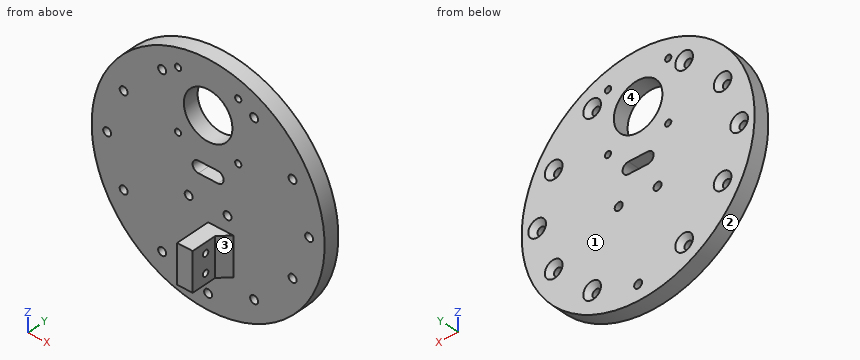
from build123d import *

# Parameters (mm, degrees)
SKETCH1_R                                           = 60
BOSS_EXTRUDE1_DEPTH                                 = 8
SKETCH2_R                                           = 12.5
SKETCH2_R_2                                         = 1.6
CUT_EXTRUDE1_DEPTH                                  = 86.229103011
SKETCH3_R                                           = 2.05
CUT_EXTRUDE2_DEPTH                                  = 86.229103011
CIRPATTERN1_COUNT                                   = 4
SKETCH4_R                                           = 2.05
CUT_EXTRUDE3_DEPTH                                  = 86.229103011
SKETCH5_R                                           = 2.05
CUT_EXTRUDE4_DEPTH                                  = 86.229103011
SKETCH6_W                                           = 8
SKETCH6_H                                           = 20
BOSS_EXTRUDE2_DEPTH                                 = 18
CHAMFER1_SIZE                                       = 5
SKETCH7_R                                           = 1.6
CUT_EXTRUDE5_DEPTH                                  = 93.455394651
CSK_FOR_M4_COUNTERSUNK_FLAT_HEAD_SCREW1_D           = 4.1
CSK_FOR_M4_COUNTERSUNK_FLAT_HEAD_SCREW1_DEPTH       = 7.999
CSK_FOR_M4_COUNTERSUNK_FLAT_HEAD_SCREW1_CSINK_D     = 9.1
CSK_FOR_M4_COUNTERSUNK_FLAT_HEAD_SCREW1_CSINK_ANGLE = 90
CSK_FOR_M4_COUNTERSUNK_FLAT_HEAD_SCREW1_TIP         = 1.231764269


with BuildPart() as part:
    # Sketch1 → Boss-Extrude1 (new body)
    with BuildSketch(Plane(origin=(0, 0, 0), x_dir=(1, 0, 0), z_dir=(0, 1, 0))):
        with Locations(Location((0, 0, 0), (0, 0, 270))):
            Circle(SKETCH1_R)
    extrude(amount=BOSS_EXTRUDE1_DEPTH)

    # Sketch2 → Cut-Extrude1 (cut, through all)
    with BuildSketch(Plane(origin=(0, 8, 0), x_dir=(1, 0, 0), z_dir=(0, 1, 0))):
        with Locations(Location((0, -33, 0), (0, 0, 270))):
            Circle(SKETCH2_R)
        with Locations(Location((-15.5, -48.5, 0), (0, 0, 270))):
            Circle(SKETCH2_R_2)
        with Locations(Location((15.5, -48.5, 0), (0, 0, 270))):
            Circle(SKETCH2_R_2)
        with Locations(Location((15.5, -17.5, 0), (0, 0, 270))):
            Circle(SKETCH2_R_2)
        with Locations(Location((-15.5, -17.5, 0), (0, 0, 270))):
            Circle(SKETCH2_R_2)
    extrude(amount=-CUT_EXTRUDE1_DEPTH, mode=Mode.SUBTRACT)

    # Sketch3 → Cut-Extrude2 (cut, through all)
    with BuildSketch(Plane(origin=(0, 8, 0), x_dir=(1, 0, 0), z_dir=(0, 1, 0))):
        with Locations(Location((-43.487067043, -23.68807717, 0), (0, 0, 270))):
            Circle(SKETCH3_R)
        with Locations(Location((-23.68807717, -43.487067043, 0), (0, 0, 270))):
            Circle(SKETCH3_R)
    cut_extrude2 = extrude(amount=-CUT_EXTRUDE2_DEPTH, mode=Mode.SUBTRACT)

    # CirPattern1: Cut-Extrude2 ×4 about axis
    cirpattern1_axis = Axis((0, 0, 0), (0, 1, 0))
    for i in range(1, CIRPATTERN1_COUNT):
        add(cut_extrude2.rotate(cirpattern1_axis, i * 360 / CIRPATTERN1_COUNT), mode=Mode.SUBTRACT)

    # Sketch4 → Cut-Extrude3 (cut, through all)
    with BuildSketch(Plane(origin=(0, 8, 0), x_dir=(1, 0, 0), z_dir=(0, 1, 0))):
        with Locations(Location((-52, 0, 0), (0, 0, 270))):
            Circle(SKETCH4_R)
        with Locations(Location((52, 0, 0), (0, 0, 270))):
            Circle(SKETCH4_R)
        with Locations(Location((0, 52, 0), (0, 0, 270))):
            Circle(SKETCH4_R)
    extrude(amount=-CUT_EXTRUDE3_DEPTH, mode=Mode.SUBTRACT)

    # Sketch5 → Cut-Extrude4 (cut, through all)
    with BuildSketch(Plane(origin=(0, 8, 0), x_dir=(1, 0, 0), z_dir=(0, 1, 0))):
        with Locations(Location((-10, 10, 0), (0, 0, 270))):
            Circle(SKETCH5_R)
        with Locations(Location((10, 10, 0), (0, 0, 270))):
            Circle(SKETCH5_R)
        with BuildLine():
            Line((-5, -3), (5, -3))
            ThreePointArc((5, -3), (8, -6), (5, -9))
            Line((5, -9), (-5, -9))
            ThreePointArc((-5, -9), (-8, -6), (-5, -3))
        make_face()
    extrude(amount=-CUT_EXTRUDE4_DEPTH, mode=Mode.SUBTRACT)

    # Sketch6 → Boss-Extrude2 (add)
    with BuildSketch(Plane.XZ):
        with Locations((4, -28)):
            Rectangle(SKETCH6_W, SKETCH6_H)
    extrude(amount=BOSS_EXTRUDE2_DEPTH)

    # Chamfer1
    chamfer1_edges = [part.edges().sort_by_distance(p)[0] for p in [
        (8, 0, -28),
    ]]
    chamfer(chamfer1_edges, length=CHAMFER1_SIZE)

    # Sketch7 → Cut-Extrude5 (cut, through all)
    with BuildSketch(Plane(origin=(8, 0, 0), x_dir=(0, 0, -1), z_dir=(1, 0, 0))):
        with Locations((23.25, -10.5)):
            Circle(SKETCH7_R)
        with Locations((32.75, -10.5)):
            Circle(SKETCH7_R)
    extrude(amount=-CUT_EXTRUDE5_DEPTH, mode=Mode.SUBTRACT)

    # CSK for M4 Countersunk Flat Head Screw1
    with Locations(Plane(origin=(-52, 8, 0), x_dir=(0, 0, 1), z_dir=(0, 1, 0))):
        with Locations((0, 0), (23.68807717, 8.512932957), (43.487067043, 28.31192283), (43.487067043, 75.68807717), (23.68807717, 95.487067043), (0, 104), (-23.68807717, 95.487067043), (-43.487067043, 75.68807717), (-43.487067043, 28.31192283), (-23.68807717, 8.512932957)):
            CounterSinkHole(CSK_FOR_M4_COUNTERSUNK_FLAT_HEAD_SCREW1_D / 2, CSK_FOR_M4_COUNTERSUNK_FLAT_HEAD_SCREW1_CSINK_D / 2, depth=CSK_FOR_M4_COUNTERSUNK_FLAT_HEAD_SCREW1_DEPTH, counter_sink_angle=CSK_FOR_M4_COUNTERSUNK_FLAT_HEAD_SCREW1_CSINK_ANGLE)
            with Locations((0, 0, -(CSK_FOR_M4_COUNTERSUNK_FLAT_HEAD_SCREW1_DEPTH + CSK_FOR_M4_COUNTERSUNK_FLAT_HEAD_SCREW1_TIP / 2))):  # 118° drill point
                Cone(0, CSK_FOR_M4_COUNTERSUNK_FLAT_HEAD_SCREW1_D / 2, CSK_FOR_M4_COUNTERSUNK_FLAT_HEAD_SCREW1_TIP, mode=Mode.SUBTRACT)


solid = part.part
Geometry: final body of the model. Coordinates: model frame, mm. Face numbers are marked on the shaded views. Give positions to 0.01 mm unless a question says otherwise; leave off trailing zeros. Loops run counter-clockwise (first coordinate to the right, second up) from the corner with the lowest first, then second, coordinate; pieces in that order, holes last. Notation, with made-up numbers: (26, 9.25) - (83, 9.25) arc R20 ccw to (83, 43.25) - close; hole circle Ø10 at (26, 56). An arc over 180 degrees is marked (long way). One line per question, with ' | ' between items. Start each with the question number.
(1) Section query D-D on z = -10. Return loops of the section in (x, y), then the cut area to 3 significant figures.
(2) Contact query for flat-ended pins moving along their axis: pin 1 (9 mm diameter, centred on x = 1, y = 4.5, fed in from +Z); pin 2 (10.5 mm diameter, centred on x = 4.5, y = -7, fed in from -Z); pin 3 (8 mm diameter, centred on x = -12, z = 41, fed in from -Y); pin 4 (12 mm diameter, centred on x = -15, y = -5, fed in from -Z). Output: stop coordinate, or through.
(3) Ray query, line 1 (X direction, y = 2.75, z = -10); line 2 (X direction, y = 6.75, z = -1); line 3 (Y direction, x = 35, z = 23.5). Return the intervals inside material, ascending. Write a range as from..to.
(4) Section query B-B on z = 33. Return loops of the section in (x, y), then the cut area to 3 significant figures.
(5) Section query C-C on x = 10. Return loops of the section in (y, z), then the cut area to 3 significant figures.
(6) Pull-direction query (X, two-part tool) for the marked faces 1, 2, 3 and 4; classes: released by +X, released by -X, zero draft, split by the parting line, or undercut.
(7) Section query A-A on y = -10.5. Return loops of the section in (x, z).
The answers:
1) outline: (-59.16, 0) - (-12.05, 0) - (-12.05, 8) - (-59.16, 8) - close; (-7.95, 0) - (7.95, 0) - (7.95, 8) - (-7.95, 8) - close; (12.05, 0) - (59.16, 0) - (59.16, 8) - (12.05, 8) - close | area: 881 mm2
2) pin 1: z = 60 | pin 2: z = -38 | pin 3: y = 0 | pin 4: z = -58.85
3) line 1: -59.16..-12.05, -7.95..7.95, 12.05..59.16 | line 2: -59.99..-55.14, -48.86..48.86, 55.14..59.99 | line 3: 0..8
4) outline: (-50.11, 0) - (-12.5, 0) - (-12.5, 8) - (-50.11, 8) - close; (12.5, 0) - (50.11, 0) - (50.11, 8) - (12.5, 8) - close | area: 602 mm2
5) outline: (-3, -38) - (0, -38) - (0, -59.16) - (8, -59.16) - (8, -12.05) - (0, -12.05) - (0, -18) - (-3, -18) - close; (0, -7.95) - (8, -7.95) - (8, 25.5) - (0, 25.5) - close; (0, 40.5) - (8, 40.5) - (8, 59.16) - (0, 59.16) - close | area: 854 mm2
6) face 1: zero draft | face 2: split by the parting line | face 3: released by +X | face 4: undercut
7) outline: (0, -38) - (8, -38) - (8, -34.35) - (0, -34.35) - close; (0, -31.15) - (8, -31.15) - (8, -24.85) - (0, -24.85) - close; (0, -21.65) - (8, -21.65) - (8, -18) - (0, -18) - close
